Work out the finished part from the listing and answer in its coordinate system (mm). A direction names the side the tool comes from. Coordinates: 2 decimals unless noted, no trailing zeros. Write each loop counter-clockwise with the first axis right and the second up, starting at its lowest first coordinate (ties: lowest second). Pieces come first, ordered by that corner, then holes. Notation, with made-up numbers: (56, 7.5) - (102, 7.5) arc R10 cw to (102, 12.5) - close; hole circle Ø1 at (1.25, 9). An arc over 180 degrees is marked (long way). One line per item, written item: value.
```python
from build123d import *

# Parameters (mm, degrees)
BOSS_EXTRUDE1_DEPTH         = 6.35
FILLET1_R                   = 1
TAP_DRILL_FOR_M2X0_4_TAP1_D = 1.6
SKETCH7_R                   = 0.8
CUT_EXTRUDE1_DEPTH          = 7.35
FILLET1_OF_MIRROR1_R        = 1
SKETCH6_W                   = 25
SKETCH6_H                   = 6.35
BOSS_EXTRUDE2_DEPTH         = 10
FILLET2_R                   = 3
FILLET2_OF_MIRROR2_R        = 3
SKETCH8_R                   = 2
CUT_EXTRUDE2_DEPTH          = 10


with BuildPart() as part:
    # Sketch1 → Boss-Extrude1 (new body)
    with BuildSketch(Plane(origin=(0, 0, 0), x_dir=(1, 0, 0), z_dir=(0, 1, 0))):
        Polygon((10, 10), (10, 36), (0, 46), (0, 0), align=None)
        Polygon((10, 36), (80, 36), (90, 46), (0, 46), align=None)
        Polygon((80, 10), (90, 0), (0, 0), (10, 10), align=None)
        Polygon((80, 10), (80, 36), (90, 46), (90, 0), align=None)
    boss_extrude1 = extrude(amount=BOSS_EXTRUDE1_DEPTH)

    # Fillet1
    fillet1_edges = [part.edges().sort_by_distance(p)[0] for p in [
        (10, 3.175, -10),
        (80, 3.175, -10),
        (80, 3.175, -36),
        (10, 3.175, -36),
    ]]
    fillet(fillet1_edges, radius=FILLET1_R)

    # Tap Drill for M2x0.4 Tap1 (through all)
    with Locations(Plane(origin=(0, 6.35, 0), x_dir=(1, 0, 0), z_dir=(0, 1, 0))):
        with Locations((85, 5), (5, 5)):
            tap_drill_for_m2x0_4_tap1 = Hole(TAP_DRILL_FOR_M2X0_4_TAP1_D / 2)

    # Sketch7 → Cut-Extrude1 (cut, through all)
    with BuildSketch(Plane(origin=(0, 6.35, 0), x_dir=(1, 0, 0), z_dir=(0, 1, 0))):
        with Locations((85, 23)):
            Circle(SKETCH7_R)
        with Locations((45, 5)):
            Circle(SKETCH7_R)
        with Locations((5, 23)):
            Circle(SKETCH7_R)
    cut_extrude1 = extrude(amount=-CUT_EXTRUDE1_DEPTH, mode=Mode.SUBTRACT)

    # Mirror1: Boss-Extrude1, Tap Drill for M2x0.4 Tap1 across plane
    add(boss_extrude1.mirror(Plane(origin=(0, 0, -46), x_dir=(1, 0, 0), z_dir=(0, 0, -1))))
    add(tap_drill_for_m2x0_4_tap1.mirror(Plane(origin=(0, 0, -46), x_dir=(1, 0, 0), z_dir=(0, 0, -1))), mode=Mode.SUBTRACT)

    # Fillet1 of Mirror1
    fillet1_of_mirror1_edges = [part.edges().sort_by_distance(p)[0] for p in [
        (10, 3.175, -82),
        (80, 3.175, -82),
        (80, 3.175, -56),
        (10, 3.175, -56),
    ]]
    fillet(fillet1_of_mirror1_edges, radius=FILLET1_OF_MIRROR1_R)

    # Sketch6 → Boss-Extrude2 (add)
    with BuildSketch(Plane(origin=(90, 0, 0), x_dir=(0, 0, -1), z_dir=(1, 0, 0))):
        with Locations((46, 3.175)):
            Rectangle(SKETCH6_W, SKETCH6_H)
    boss_extrude2 = extrude(amount=BOSS_EXTRUDE2_DEPTH)

    # Fillet2
    fillet2_edges = [part.edges().sort_by_distance(p)[0] for p in [
        (100, 3.175, -58.5),
        (100, 3.175, -33.5),
    ]]
    fillet(fillet2_edges, radius=FILLET2_R)

    # Mirror2: Boss-Extrude2 across plane
    add(boss_extrude2.mirror(Plane.ZY.offset(-45)))

    # Fillet2 of Mirror2
    fillet2_of_mirror2_edges = [part.edges().sort_by_distance(p)[0] for p in [
        (-10, 3.175, -58.5),
        (-10, 3.175, -33.5),
    ]]
    fillet(fillet2_of_mirror2_edges, radius=FILLET2_OF_MIRROR2_R)

    # Mirror3: Cut-Extrude1 across plane
    add(cut_extrude1.mirror(Plane(origin=(0, 0, -46), x_dir=(1, 0, 0), z_dir=(0, 0, -1))), mode=Mode.SUBTRACT)

    # Sketch8 → Cut-Extrude2 (cut)
    with BuildSketch(Plane(origin=(0, 0, 0), x_dir=(-1, 0, 0), z_dir=(0, -1, 0))):
        with Locations((-45, 46)):
            Circle(SKETCH8_R)
        with Locations((-85, 46)):
            Circle(SKETCH8_R)
        with Locations((-5, 46)):
            Circle(SKETCH8_R)
    extrude(amount=-CUT_EXTRUDE2_DEPTH, mode=Mode.SUBTRACT)


solid = part.part
```
Item 1: Section A-A, the plane x = 69.5 is taken. Determine the outline of the cut face in (y, z), then the cut area to 3 significant figures.
Evaluation:
outline: (0, -92) - (6.35, -92) - (6.35, -82) - (0, -82) - close; (0, -56) - (6.35, -56) - (6.35, -36) - (0, -36) - close; (0, -10) - (6.35, -10) - (6.35, 0) - (0, 0) - close
area: 254 mm2
Item 2: Consider probe 1 along Z at (x, y) = (45, 3.5); probe 2 along Z at (x, y) = (5, 5); probe 3 along X at (y, z) = (2.5, -46). Determine where each line is inside the solid, lowest interval first.
Evaluation:
probe 1: z = -92 to -87.8, -86.2 to -82, -56 to -48, -44 to -36, -10 to -5.8, -4.2 to 0
probe 2: z = -92 to -87.8, -86.2 to -69.8, -68.2 to -48, -44 to -23.8, -22.2 to -5.8, -4.2 to 0
probe 3: x = -10 to 3, 7 to 43, 47 to 83, 87 to 100
Item 3: Given pin 1 (3 mm diameter, centred on x = -3.5, y = 4, fed in from -Z); pin 2 (2 mm diameter, centred on x = 5, z = -5, fed in from -Y); pin 3 (3 mm diameter, centred on y = 4, z = -12.5, fed in from +X), each flat-ended and moving along its own axis, determine where each tip first touches the part or whether it passes through.
Evaluation:
pin 1: stops at z = -58.5
pin 2: stops at y = 0
pin 3: stops at x = 90
Item 4: Determine the mould class of faces 5 (the face through (99.1, 3.22, -57.64)), 6 (the face through (45, 3, -36)), 7 (the face through (99.1, 3.22, -34.36)) for opening direction Z: +Z half, -Z half, draft (parallel to the pull), parting line (faces both ways), or undercut.
Evaluation:
face 5: -Z half
face 6: undercut
face 7: +Z half
Item 5: Section C-C, the plane y = 4.25 is taken. Give the number of separate pieces and of enclosed holes in the cut face, then the cut area to 3 significant figures.
Evaluation:
separate pieces: 1
enclosed holes: 15
area: 5,080 mm2
Item 6: Which of the six approach directions +Z, -Z, +X, -X, +Y, -Y give full straight-line access (tool end or side, diameter ignored) to faces 1 (the face through (0, 3, -17)), 2 (the face through (-3, 3, -58.5)), 3 (the face through (80, 3, -69)), 4 (the face through (90, 3, -17))?
Evaluation:
face 1: +Z, -X, +Y, -Y
face 2: -Z, -X, +Y, -Y
face 3: +Y, -Y
face 4: +Z, +X, +Y, -Y
Item 7: Section B-B, the plane z = -29 is taken. Determine the outline of the cut face in (x, y), then the cut area to 3 significant figures.
Evaluation:
outline: (0, 0) - (10, 0) - (10, 6.35) - (0, 6.35) - close; (80, 0) - (90, 0) - (90, 6.35) - (80, 6.35) - close
area: 127 mm2
